Design review of the part built by this model. Coordinates are the model's own, in mm. A direction names the side the tool comes from. Coordinates: 2 decimals unless noted, no trailing zeros. Loops run counter-clockwise (first coordinate to the right, second up) from the corner with the lowest first, then second, coordinate; pieces in that order, holes last.
Q1. Add section C-C on y = -11.5. Give the boundary of the cut face in (x, z) (3 decimals), and give its area (3 significant figures).
Q2. For P1, Ø8, axis at x = 18, y = 0.5, coming from the +Z side (3 decimals); P2, Ø1.5, axis at x = -12, y = 1.5, coming from the -Z side; P3, Ø10, axis at x = -19, z = 12, coming from the -Y side, all flat-tipped, find the tip position at first contact; note any pin that passes through.
Q3. Wall thickness on probe 1 along X at (y, z) = (-12, 19); probe 2 along Z at (x, y) = (-22, 1) (3 decimals); probe 3 along X at (y, z) = (-1, 3): over which ranges is each line inside the solid? List them lowest first.
Q4. Add section B-B on z = 34. Give the boundary of the cut face in (x, y) (3 decimals), and give its area (3 significant figures).
Q5. Add section D-D on z = 22. Give the boundary of the cut face in (x, y) (3 decimals), and give its area (3 significant figures).
Q6. Draft analysis for pull direction X (two halves, no side actions). For faces 1 (the face through (30.226, -7, 16)), 2 (the face through (33.401, -4, 20)), 3 (the face through (-32.146, -0.222, 1.191)), state which applies: released by +X, released by -X, zero draft, split by the parting line, or undercut.
Q7. Machinability: for faces 4 (the face through (0, 4, 0)), 5 (the face through (0, 4, 3.175)), which of the approach directions +Z, -Z, +X, -X, +Y, -Y give a long, thin tool a straight path to every point of the face, cutting with its end or side? Answer none if there is none.
```python
from build123d import *

# Parameters (mm, degrees)
SKETCH2_W                    = 60.452
SKETCH2_H                    = 31.75
BASE_FLANGE1_DEPTH           = 3.175
EDGE_FLANGE1_STRIP_W         = 14.7
EDGE_FLANGE1_STRIP_H         = 3.175
EDGE_FLANGE1_STRIP_CUT_DEPTH = 31.75
EDGE_FLANGE1_DEPTH           = 31.75
CUT_EXTRUDE1_START           = -3.175
CUT_EXTRUDE1_DEPTH           = 83.39755521
M6_CLEARANCE_HOLE1_D         = 6.6


# Sheet-metal steps are written as plain solids
with BuildPart() as part:
    # Sketch2 → Base-Flange1 (new body)
    with BuildSketch(Plane.XY):
        Rectangle(SKETCH2_W, SKETCH2_H)
    extrude(amount=BASE_FLANGE1_DEPTH)

    # Edge-Flange1 strip (across the edge) → Edge-Flange1 strip cut (cut)
    with BuildSketch(Plane(origin=(30.226, -15.875, 3.175), x_dir=(-1, 0, 0), z_dir=(0, 1, 0))):
        with Locations((-6.35, -1.5875)):
            Rectangle(EDGE_FLANGE1_STRIP_W, EDGE_FLANGE1_STRIP_H)
    edge_flange1_strip_cut = extrude(amount=EDGE_FLANGE1_STRIP_CUT_DEPTH, mode=Mode.SUBTRACT)

    # Edge-Flange1 section (across the edge) → Edge-Flange1 (add)
    with BuildSketch(Plane(origin=(30.226, -15.875, 3.175), x_dir=(-1, 0, 0), z_dir=(0, 1, 0))):
        with BuildLine():
            Line((-3.175, 1), (-3.175, 41.275))
            Line((-3.175, 41.275), (0, 41.275))
            Line((0, 41.275), (0, 1))
            ThreePointArc((0, 1), (0.292893219, 0.292893219), (1, 0))
            Line((1, 0), (1, -3.175))
            ThreePointArc((1, -3.175), (-1.952170811, -1.952170811), (-3.175, 1))
        make_face()
    edge_flange1 = extrude(amount=EDGE_FLANGE1_DEPTH)

    # Sketch10 → Cut-Extrude1 (cut)
    with BuildSketch(Plane(origin=(33.401, 0, 0), x_dir=(0, 0, -1), z_dir=(1, 0, 0)).offset(CUT_EXTRUDE1_START)):
        Polygon((-4.175, 15.875), (-44.45, -15.875), (-44.45, 15.875), align=None)
    cut_extrude1 = extrude(amount=CUT_EXTRUDE1_DEPTH, mode=Mode.SUBTRACT)

    # Mirror1: Edge-Flange1 strip cut, Edge-Flange1, Cut-Extrude1 across plane
    add(edge_flange1_strip_cut.mirror(Plane(origin=(0, 0, 0), x_dir=(0, 0, 1), z_dir=(1, 0, 0))), mode=Mode.SUBTRACT)
    add(edge_flange1.mirror(Plane(origin=(0, 0, 0), x_dir=(0, 0, 1), z_dir=(1, 0, 0))))
    add(cut_extrude1.mirror(Plane(origin=(0, 0, 0), x_dir=(0, 0, 1), z_dir=(1, 0, 0))), mode=Mode.SUBTRACT)

    # M6 Clearance Hole1 (through all)
    with Locations(Plane.XY.offset(3.175)):
        with Locations((-1.5146, 0)):
            Hole(M6_CLEARANCE_HOLE1_D / 2)


solid = part.part
```
Entries:
1. outline: (-33.401, 4.175) arc R4.175 ccw to (-29.226, 0) - (29.226, 0) arc R4.175 ccw to (33.401, 4.175) - (33.401, 38.9) - (30.226, 38.9) - (30.226, 4.175) arc R1 cw to (29.226, 3.175) - (-29.226, 3.175) arc R1 cw to (-30.226, 4.175) - (-30.226, 38.9) - (-33.401, 38.9) - close
1. area: 432 mm2
2. P1: stops at z = 3.175
2. P2: stops at z = 0
2. P3: passes through
3. probe 1: x = -33.4 to -30.23, 30.23 to 33.4
3. probe 2: z = 0 to 3.175
3. probe 3: x = -33.23 to -4.66, 1.63 to 33.23
4. outline: (-33.401, -15.875) - (-30.226, -15.875) - (-30.226, -7.637) - (-33.401, -7.637) - close; (30.226, -15.875) - (33.401, -15.875) - (33.401, -7.637) - (30.226, -7.637) - close
4. area: 52.3 mm2
5. outline: (-33.401, -15.875) - (-30.226, -15.875) - (-30.226, 1.823) - (-33.401, 1.823) - close; (30.226, -15.875) - (33.401, -15.875) - (33.401, 1.823) - (30.226, 1.823) - close
5. area: 112 mm2
6. face 1: undercut
6. face 2: released by +X
6. face 3: released by -X
7. face 4: -Z, +X, -X, +Y, -Y
7. face 5: +Z, +Y, -Y
